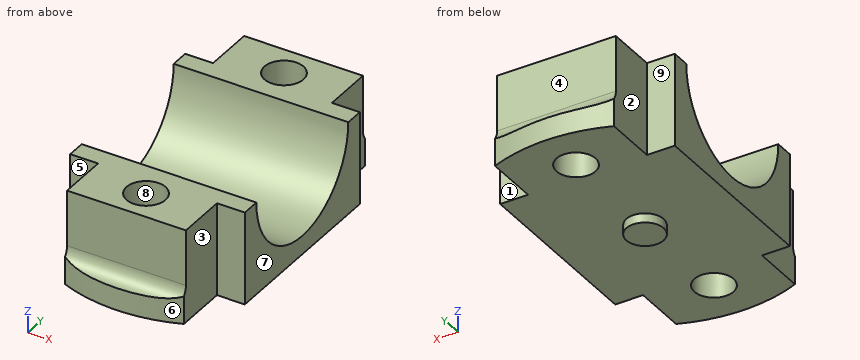
from build123d import *

# Parameters (mm, degrees)
SKETCH1_R           = 10.5
SKETCH1_W           = 94
SKETCH1_H           = 80
BOSS_EXTRUDE1_DEPTH = 50
CUT_EXTRUDE1_DEPTH  = 137.238761004
SKETCH3_R           = 10
BOSS_EXTRUDE2_DEPTH = 5


with BuildPart() as part:
    # Sketch1 → Boss-Extrude1 (new body)
    # profile 1 of 5: a face of its own
    with BuildSketch(Plane.XY):
        with BuildLine():
            Line((32, 67.830671528), (32, 78.74642849))
            ThreePointArc((32, 78.74642849), (0, 85), (-32, 78.74642849))
            Line((-32, 78.74642849), (-32, 67.830671528))
            ThreePointArc((-32, 67.830671528), (0, 75), (32, 67.830671528))
        make_face()
    # profile 2 of 5: a face of its own
    with BuildSketch(Plane.XY):
        with BuildLine():
            Line((32, 67.830671528), (32, 50))
            Line((32, 50), (47, 50))
            Line((47, 50), (47, 40))
            Line((47, 40), (-47, 40))
            Line((-47, 40), (-47, 50))
            Line((-47, 50), (-32, 50))
            Line((-32, 50), (-32, 67.830671528))
            ThreePointArc((-32, 67.830671528), (0, 75), (32, 67.830671528))
        make_face()
        with Locations((0, 60)):
            Circle(SKETCH1_R, mode=Mode.SUBTRACT)
    # profile 3 of 5: a face of its own
    with BuildSketch(Plane.XY):
        Rectangle(SKETCH1_W, SKETCH1_H)
    # profile 4 of 5: a face of its own
    with BuildSketch(Plane.XY):
        with BuildLine():
            Line((-32, -67.830671528), (-32, -50))
            Line((-32, -50), (-47, -50))
            Line((-47, -50), (-47, -40))
            Line((-47, -40), (47, -40))
            Line((47, -40), (47, -50))
            Line((47, -50), (32, -50))
            Line((32, -50), (32, -67.830671528))
            ThreePointArc((32, -67.830671528), (0, -75), (-32, -67.830671528))
        make_face()
        with Locations((0, -60)):
            Circle(SKETCH1_R, mode=Mode.SUBTRACT)
    # profile 5 of 5: a face of its own
    with BuildSketch(Plane.XY):
        with BuildLine():
            Line((-32, -67.830671528), (-32, -78.74642849))
            ThreePointArc((-32, -78.74642849), (0, -85), (32, -78.74642849))
            Line((32, -78.74642849), (32, -67.830671528))
            ThreePointArc((32, -67.830671528), (0, -75), (-32, -67.830671528))
        make_face()
    extrude(amount=BOSS_EXTRUDE1_DEPTH)

    # Sketch2 → Cut-Extrude1 (cut, through all)
    with BuildSketch(Plane(origin=(47, 0, 0), x_dir=(0, 0, -1), z_dir=(1, 0, 0))):
        with BuildLine():
            Line((-50, 40), (-50, -40))
            ThreePointArc((-50, -40), (-10, 0), (-50, 40))
        make_face()
        with BuildLine():
            Line((-50, -77), (-20, -77))
            ThreePointArc((-20, -77), (-14.343145751, -79.343145751), (-12, -85))
            Line((-12, -85), (-50, -85))
            Line((-50, -85), (-50, -77))
        make_face()
        with BuildLine():
            Line((-50, 85), (-12, 85))
            ThreePointArc((-12, 85), (-14.343145751, 79.343145751), (-20, 77))
            Line((-20, 77), (-50, 77))
            Line((-50, 77), (-50, 85))
        make_face()
    extrude(amount=-CUT_EXTRUDE1_DEPTH, mode=Mode.SUBTRACT)

    # Sketch3 → Boss-Extrude2 (add)
    with BuildSketch(Plane(origin=(0, 0, 0), x_dir=(-1, 0, 0), z_dir=(0, 0, -1))):
        with Locations(Location((0, 0, 0), (0, 0, 180))):
            Circle(SKETCH3_R)
    extrude(amount=BOSS_EXTRUDE2_DEPTH)


solid = part.part
For this review, take the finished solid that the model builds, in its own axes (mm). Face numbers are marked on the shaded views. A direction names the side the tool comes from. Round coordinates to 2 decimals unless told otherwise and drop trailing zeros. Order: outer loops, then holes, each group sorted by start corner. A loop starts at its lowest first (then second) coordinate and runs counter-clockwise, first axis right, second up. Notation, with made-up numbers: M 5.5,19 L 24.5,19 A11 cw 24.5,30 Z; hole C 26,-7.75 d9. An arc over 180 degrees is marked long. Use a Markdown table: item, result. Add a question column.
Item 1: Tool access review of the marked faces 1, 2, 3, 4 and 5: name each direction out of +Z, -Z, +X, -X, +Y, -Y from which nothing blocks a thin tool from reaching the whole face with its end or side.
Item 2: Add section D-D, the plane x = -3. Give the boundary of the cut face in (y, z).
Item 3: Mouldability with a two-part tool opening along Y and no side actions: class the marked faces 6, 7, 8 and 9 as released by +Y, released by -Y, zero draft, split by the parting line, or undercut.
Item 4: Add section C-C, the plane z = 4.5. Give the boundary of the cut face in (x, y).
Item 5: Add section A-A, the plane z = 37.5. Give the boundary of the cut face in (x, y), then the cut area to 3 significant figures.
Item 6: Add section B-B, the plane y = -60. Give the boundary of the cut face in (x, z), then the cut area to 3 significant figures.
Item 7: To check wall thickness, follow line 1 along Y through (x, z) = (0, 22.5); line 2 along Y through (x, z) = (0, 40); line 3 along Z through (x, y) = (-26.5, -1). State the ranges of each line that lie inside material, in increasing order.
Item 8: Insertion check: pin 1 (1 mm diameter, centred on x = -36.5, y = 24, fed in from +Z); pin 2 (16.5 mm diameter, centred on x = 37.5, z = 16.5, fed in from +Y); pin 3 (4.5 mm diameter, centred on x = -39.5, z = 15, fed in from +Y); pin 4 (19 mm diameter, centred on x = 0, y = -60, fed in from +Z). Each pin has a flat end and moves straight along its axis. Give the tip position at first contact, or say it passes through.
Geometry results:
| question | item | result |
|---|---|---|
| 1 | face 1 | +Z, -Z, +X, +Y |
| 1 | face 2 | +Z, -Z, -X, +Y |
| 1 | face 3 | +Z, -Z, +X, -Y |
| 1 | face 4 | +Z, +X, -X, +Y |
| 1 | face 5 | +Z, -Z, -X, -Y |
| 2 | outline | M -84.95,0 L -70.06,0 L -70.06,50 L -77,50 L -77,20 A8 cw -84.95,12 Z; M -49.94,0 L -9.54,0 L -9.54,-5 L 9.54,-5 L 9.54,0 L 49.94,0 L 49.94,50 L 40,50 A40 cw -40,50 L -49.94,50 Z; M 70.06,0 L 84.95,0 L 84.95,12 A8 cw 77,20 L 77,50 L 70.06,50 Z |
| 3 | face 6 | released by -Y |
| 3 | face 7 | zero draft |
| 3 | face 8 | undercut |
| 3 | face 9 | released by +Y |
| 4 | outline | M -47,-50 L -32,-50 L -32,-78.75 A85 ccw 32,-78.75 L 32,-50 L 47,-50 L 47,50 L 32,50 L 32,78.75 A85 ccw -32,78.75 L -32,50 L -47,50 Z; hole C 0,-60 d21; hole C 0,60 d21 |
| 5 | outline | M -47,-50 L -32,-50 L -32,-77 L 32,-77 L 32,-50 L 47,-50 L 47,-38 L -47,-38 Z; M -47,38 L 47,38 L 47,50 L 32,50 L 32,77 L -32,77 L -32,50 L -47,50 Z; hole C 0,-60 d21; hole C 0,60 d21 |
| 5 | area | 5,020 mm² |
| 6 | outline | M -32,0 L -10.5,0 L -10.5,50 L -32,50 Z; M 10.5,0 L 32,0 L 32,50 L 10.5,50 Z |
| 6 | area | 2,150 mm² |
| 7 | line 1 | y = -77 to -70.5, -49.5 to -29.05, 29.05 to 49.5, 70.5 to 77 |
| 7 | line 2 | y = -77 to -70.5, -49.5 to -38.73, 38.73 to 49.5, 70.5 to 77 |
| 7 | line 3 | z = 0 to 10.01 |
| 8 | pin 1 | stops at z = 18.38 |
| 8 | pin 2 | stops at y = 79.67 |
| 8 | pin 3 | stops at y = 50 |
| 8 | pin 4 | passes through |
